Read the model definition and answer for the solid it produces. Units are mm, in the model's axes. Give positions to 0.01 mm unless a question says otherwise; leave off trailing zeros. Order: outer loops, then holes, each group sorted by start corner. A loop starts at its lowest first (then second) coordinate and runs counter-clockwise, first axis right, second up. Notation, with made-up numbers: M 75,-14.75 L 114,-14.75 A37 cw 114,23.25 Z; hole C 17.25,-37 d7. An arc over 180 degrees is marked long. One line per item, written item: value.
from build123d import *

# Parameters (mm, degrees)
SKETCH_W                           = 30
SKETCH_H                           = 20
PAD_DEPTH                          = 10
SKETCH001_R                        = 2.4975
POCKET_DEPTH                       = 10
SKETCH001_LINEARPATTERN_2_R        = 2.4975
POCKET_LINEARPATTERN_2_DEPTH       = 10
SKETCH001_LINEARPATTERN_3_R        = 2.4975
POCKET_LINEARPATTERN_3_DEPTH       = 10
LINEARPATTERN001_COUNT             = 2
LINEARPATTERN001_PITCH             = 10.01
SKETCH002_R                        = 2.4975
POCKET001_DEPTH                    = 20
SKETCH002_LINEARPATTERN002_2_R     = 2.4975
POCKET001_LINEARPATTERN002_2_DEPTH = 20
SKETCH002_LINEARPATTERN002_3_R     = 2.4975
POCKET001_LINEARPATTERN002_3_DEPTH = 20
LINEARPATTERN003_COUNT             = 1
LINEARPATTERN003_PITCH             = 0
SKETCH003_R                        = 2.4975
POCKET002_DEPTH                    = 30
SKETCH003_LINEARPATTERN004_2_R     = 2.4975
POCKET002_LINEARPATTERN004_2_DEPTH = 30
LINEARPATTERN005_COUNT             = 1
LINEARPATTERN005_PITCH             = 0


with BuildPart() as part:
    # Sketch → Pad (new body)
    with BuildSketch(Plane.XY):
        Rectangle(SKETCH_W, SKETCH_H)
    extrude(amount=PAD_DEPTH)

    # Sketch001 (on Face6 of Pad) → Pocket (cut)
    with BuildSketch(Plane.XY.offset(10)):
        with Locations((-10.005, -5.005)):
            Circle(SKETCH001_R)
    pocket = extrude(amount=-POCKET_DEPTH, mode=Mode.SUBTRACT)

    # Sketch001 LinearPattern 2 → Pocket LinearPattern 2 (cut)
    with BuildSketch(Plane(origin=(10.005, 0, 10), x_dir=(1, 0, 0), z_dir=(0, 0, 1))):
        with Locations((-10.005, -5.005)):
            Circle(SKETCH001_LINEARPATTERN_2_R)
    pocket_linearpattern_2 = extrude(amount=-POCKET_LINEARPATTERN_2_DEPTH, mode=Mode.SUBTRACT)

    # Sketch001 LinearPattern 3 → Pocket LinearPattern 3 (cut)
    with BuildSketch(Plane(origin=(20.01, 0, 10), x_dir=(1, 0, 0), z_dir=(0, 0, 1))):
        with Locations((-10.005, -5.005)):
            Circle(SKETCH001_LINEARPATTERN_3_R)
    pocket_linearpattern_3 = extrude(amount=-POCKET_LINEARPATTERN_3_DEPTH, mode=Mode.SUBTRACT)

    # LinearPattern001: Pocket, Pocket LinearPattern 2, Pocket LinearPattern 3 ×2
    with Locations(*[(0, i * LINEARPATTERN001_PITCH, 0) for i in range(1, LINEARPATTERN001_COUNT)]):
        add(pocket, mode=Mode.SUBTRACT)
        add(pocket_linearpattern_2, mode=Mode.SUBTRACT)
        add(pocket_linearpattern_3, mode=Mode.SUBTRACT)

    # Sketch002 (on Face6 of MultiTransform) → Pocket001 (cut)
    with BuildSketch(Plane.XZ.offset(10)):
        with Locations((-10.005, 4.995)):
            Circle(SKETCH002_R)
    pocket001 = extrude(amount=-POCKET001_DEPTH, mode=Mode.SUBTRACT)

    # Sketch002 LinearPattern002 2 → Pocket001 LinearPattern002 2 (cut)
    with BuildSketch(Plane(origin=(10.005, -10, 0), x_dir=(1, 0, 0), z_dir=(0, -1, 0))):
        with Locations((-10.005, 4.995)):
            Circle(SKETCH002_LINEARPATTERN002_2_R)
    pocket001_linearpattern002_2 = extrude(amount=-POCKET001_LINEARPATTERN002_2_DEPTH, mode=Mode.SUBTRACT)

    # Sketch002 LinearPattern002 3 → Pocket001 LinearPattern002 3 (cut)
    with BuildSketch(Plane(origin=(20.01, -10, 0), x_dir=(1, 0, 0), z_dir=(0, -1, 0))):
        with Locations((-10.005, 4.995)):
            Circle(SKETCH002_LINEARPATTERN002_3_R)
    pocket001_linearpattern002_3 = extrude(amount=-POCKET001_LINEARPATTERN002_3_DEPTH, mode=Mode.SUBTRACT)

    # LinearPattern003: Pocket001, Pocket001 LinearPattern002 2, Pocket001 LinearPattern002 3 ×1
    with Locations(*[(0, 0, i * LINEARPATTERN003_PITCH) for i in range(1, LINEARPATTERN003_COUNT)]):
        add(pocket001, mode=Mode.SUBTRACT)
        add(pocket001_linearpattern002_2, mode=Mode.SUBTRACT)
        add(pocket001_linearpattern002_3, mode=Mode.SUBTRACT)

    # Sketch003 (on Face2 of MultiTransform001) → Pocket002 (cut)
    with BuildSketch(Plane(origin=(-15, 0, 0), x_dir=(0, -1, 0), z_dir=(-1, 0, 0))):
        with Locations((-5.005, 4.995)):
            Circle(SKETCH003_R)
    pocket002 = extrude(amount=-POCKET002_DEPTH, mode=Mode.SUBTRACT)

    # Sketch003 LinearPattern004 2 → Pocket002 LinearPattern004 2 (cut)
    with BuildSketch(Plane(origin=(-15, -10.01, 0), x_dir=(0, -1, 0), z_dir=(-1, 0, 0))):
        with Locations((-5.005, 4.995)):
            Circle(SKETCH003_LINEARPATTERN004_2_R)
    pocket002_linearpattern004_2 = extrude(amount=-POCKET002_LINEARPATTERN004_2_DEPTH, mode=Mode.SUBTRACT)

    # LinearPattern005: Pocket002, Pocket002 LinearPattern004 2 ×1
    with Locations(*[(0, 0, i * LINEARPATTERN005_PITCH) for i in range(1, LINEARPATTERN005_COUNT)]):
        add(pocket002, mode=Mode.SUBTRACT)
        add(pocket002_linearpattern004_2, mode=Mode.SUBTRACT)


solid = part.part
1) Consider probe 1 along X at (y, z) = (5, 1.5); probe 2 along Y at (x, z) = (0, 7.6); probe 3 along Z at (x, y) = (0, 0). Determine where each line is inside the solid, lowest interval first.
Reported:
probe 1: x = -15 to -12.5, -7.51 to -2.5, 2.5 to 7.51, 12.5 to 15
probe 2: y = -10 to -7.5, -2.51 to 2.51, 7.5 to 10
probe 3: z = 0 to 2.5, 7.49 to 10
2) Find section C-C, the plane z = 1. Write down the section's boundary in (x, y) (1 decimal).
Reported:
outline: M -15,-10 L 15,-10 L 15,10 L -15,10 Z; hole C -10,-5 d5; hole C -10,5 d5; hole C 0,-5 d5; hole C 0,5 d5; hole C 10,-5 d5; hole C 10,5 d5
3) Find section B-B, the plane y = 2. Write down the section's boundary in (x, z) (1 decimal), plus the area to 3 significant figures.
Reported:
outline: M -15,0 L 15,0 L 15,10 L -15,10 Z; hole C -10,5 d5; hole C 0,5 d5; hole C 10,5 d5
area: 241 mm^2
4) Find section A-A, the plane x = 0. Write down the section's boundary in (y, z).
Reported:
outline: M -10,0 L -7.5,0 L -7.5,2.5 L -10,2.5 Z; M -10,7.49 L -7.5,7.49 L -7.5,10 L -10,10 Z; M -2.51,0 L 2.51,0 L 2.51,2.5 L -2.51,2.5 Z; M -2.51,7.49 L 2.51,7.49 L 2.51,10 L -2.51,10 Z; M 7.5,0 L 10,0 L 10,2.5 L 7.5,2.5 Z; M 7.5,7.49 L 10,7.49 L 10,10 L 7.5,10 Z
5) Determine the mould class of faces 1 (the face through (-15, 0, 5)), 2 (the face through (0, 0, 10)), 3 (the face through (-1.841, 6.693, 8.763)) for opening direction X: +X half, -X half, draft (parallel to the pull), parting line (faces both ways), or undercut.
Reported:
face 1: -X half
face 2: draft
face 3: undercut
6) Find section D-D, the plane y = 5.75. Count the separate pieces of the cut face and the enclosed holes in it, plus the area to 3 significant figures.
Reported:
separate pieces: 8
enclosed holes: 0
area: 82.1 mm^2
